```python
from build123d import *

# Parameters (mm, degrees)
SKETCH1_W           = 21
SKETCH1_H           = 21
SKETCH1_R           = 1.5
BOSS_EXTRUDE1_DEPTH = 5
FILLET1_R           = 0.5


with BuildPart() as part:
    # Sketch1 → Boss-Extrude1 (new body)
    with BuildSketch(Plane.XY):
        Rectangle(SKETCH1_W, SKETCH1_H)
        with Locations((-5.000000296, 5.000000296)):
            Circle(SKETCH1_R, mode=Mode.SUBTRACT)
        with Locations((4.999999704, 4.999999704)):
            Circle(SKETCH1_R, mode=Mode.SUBTRACT)
        with Locations((5.000000296, -5.000000296)):
            Circle(SKETCH1_R, mode=Mode.SUBTRACT)
        with Locations((-4.999999704, -4.999999704)):
            Circle(SKETCH1_R, mode=Mode.SUBTRACT)
        with Locations((0, 7)):
            Circle(SKETCH1_R, mode=Mode.SUBTRACT)
        with Locations((7, 0)):
            Circle(SKETCH1_R, mode=Mode.SUBTRACT)
        with Locations((-7, 0)):
            Circle(SKETCH1_R, mode=Mode.SUBTRACT)
        with Locations((0, -7)):
            Circle(SKETCH1_R, mode=Mode.SUBTRACT)
    extrude(amount=BOSS_EXTRUDE1_DEPTH)

    # Fillet1
    fillet1_edges = [part.edges().sort_by_distance(p)[0] for p in [
        (-10.5, 0, 5),
        (0, -10.5, 5),
        (10.5, 0, 5),
        (0, -10.5, 0),
        (-10.5, 0, 0),
        (0, 10.5, 0),
        (10.5, 0, 0),
        (10.5, -10.5, 2.5),
        (-10.5, -10.5, 2.5),
        (-10.5, 10.5, 2.5),
        (10.5, 10.5, 2.5),
        (0, 10.5, 5),
    ]]
    fillet(fillet1_edges, radius=FILLET1_R)


solid = part.part
```
Work out the finished part from the listing and answer in its coordinate system (mm). Round coordinates to 2 decimals unless told otherwise and drop trailing zeros. Write each loop counter-clockwise with the first axis right and the second up, starting at its lowest first coordinate (ties: lowest second). Pieces come first, ordered by that corner, then holes.
1) Determine the mould class of faces 1 (the face through (0, 10.5, 2)), 2 (the face through (-10.5, 0, 2)), 3 (the face through (4.805, -3.513, 2.465)) for opening direction Y: pulls with the +Y half, pulls with the -Y half, needs draft (parallel to the pull), parting line crosses it, or undercut.
2) A cutting plane is placed at A-A on x = 0. Determine the outline of the cut face in (y, z).
3) A cutting plane is placed at C-C on x = 7. Determine the outline of the cut face in (y, z).
4) Consider probe 1 along Y at (x, z) = (0.5, 2.3); probe 2 along Y at (x, z) = (-4, 2); probe 3 along Y at (x, z) = (6, 3.15). Determine where each line is inside the solid, lowest interval first.
5) A flat-ended cylindrical pin translates along its axis: P1, Ø4, axis at x = 7, y = 0, coming from the -Z side. Find the tip coordinate at first contact, or state that the pin passes through.
6) A cutting plane is placed at B-B on y = -5. Determine the outline of the cut face in (x, z).
7) A cutting plane is placed at D-D on z = 3.9. Give the number of separate pieces and of enclosed holes in the cut face, and give its area (3 significant figures).
Entries:
1. face 1: pulls with the +Y half
1. face 2: needs draft
1. face 3: undercut
2. outline: (-10.5, 0.5) arc R0.5 ccw to (-10, 0) - (-8.5, 0) - (-8.5, 5) - (-10, 5) arc R0.5 ccw to (-10.5, 4.5) - close; (-5.5, 0) - (5.5, 0) - (5.5, 5) - (-5.5, 5) - close; (8.5, 0) - (10, 0) arc R0.5 ccw to (10.5, 0.5) - (10.5, 4.5) arc R0.5 ccw to (10, 5) - (8.5, 5) - close
3. outline: (-10.5, 0.5) arc R0.5 ccw to (-10, 0) - (-1.5, 0) - (-1.5, 5) - (-10, 5) arc R0.5 ccw to (-10.5, 4.5) - close; (1.5, 0) - (10, 0) arc R0.5 ccw to (10.5, 0.5) - (10.5, 4.5) arc R0.5 ccw to (10, 5) - (1.5, 5) - close
4. probe 1: y = -10.5 to -8.41, -5.59 to 5.59, 8.41 to 10.5
4. probe 2: y = -10.5 to -6.12, -3.88 to 3.88, 6.12 to 10.5
4. probe 3: y = -10.5 to -6.12, -3.88 to -1.12, 1.12 to 3.88, 6.12 to 10.5
5. P1: stops at z = 0
6. outline: (-10.5, 0.5) arc R0.5 ccw to (-10, 0) - (-6.5, 0) - (-6.5, 5) - (-10, 5) arc R0.5 ccw to (-10.5, 4.5) - close; (-3.5, 0) - (3.5, 0) - (3.5, 5) - (-3.5, 5) - close; (6.5, 0) - (10, 0) arc R0.5 ccw to (10.5, 0.5) - (10.5, 4.5) arc R0.5 ccw to (10, 5) - (6.5, 5) - close
7. separate pieces: 1
7. enclosed holes: 8
7. area: 384 mm2
